Source: CAD feature listing. Evaluate the final solid. Frame: model axes, mm. Coordinates: 2 decimals unless noted, no trailing zeros. Order: outer loops, then holes, each group sorted by start corner. A loop starts at its lowest first (then second) coordinate and runs counter-clockwise, first axis right, second up. Notation, with made-up numbers: (85, 72.5) -> (134, 72.5) arc R10 cw to (134, 89.5) -> close; hole circle Ø6 at (46, -3). An arc over 180 degrees is marked (long way). Put each result on its own line as item: value.
from build123d import *

# Parameters (mm, degrees)
SKETCH1_W            = 40
SKETCH1_H            = 20
BOSS_EXTRUDE1_DEPTH  = 2
M3_CLEARANCE_HOLE1_D = 3.2
FILLET1_R            = 2


with BuildPart() as part:
    # Sketch1 → Boss-Extrude1 (new body)
    with BuildSketch(Plane.XY):
        Rectangle(SKETCH1_W, SKETCH1_H)
    extrude(amount=BOSS_EXTRUDE1_DEPTH)

    # M3 Clearance Hole1 (through all)
    with Locations(Plane.XY.offset(2)):
        with Locations((17.5, -5), (-17.5, 5), (-17.5, -5), (17.5, 5), (0, 5), (0, -5)):
            Hole(M3_CLEARANCE_HOLE1_D / 2)

    # Fillet1
    fillet1_edges = [part.edges().sort_by_distance(p)[0] for p in [
        (20, -10, 1),
        (-20, -10, 1),
        (-20, 10, 1),
        (20, 10, 1),
    ]]
    fillet(fillet1_edges, radius=FILLET1_R)


solid = part.part
1. Ray query, line 1 along Y through (x, z) = (-17.5, 1.05); line 2 along Y through (x, z) = (-0.5, 0.2); line 3 along X through (y, z) = (4.5, 0.6). Return the intervals inside material, ascending.
Numbers:
line 1: y = -10 to -6.6, -3.4 to 3.4, 6.6 to 10
line 2: y = -10 to -6.52, -3.48 to 3.48, 6.52 to 10
line 3: x = -20 to -19.02, -15.98 to -1.52, 1.52 to 15.98, 19.02 to 20
2. Cut plane A-A on x = 0. Output: boundary loops of the cut face in (y, z).
Numbers:
outline: (-10, 0) -> (-6.6, 0) -> (-6.6, 2) -> (-10, 2) -> close; (-3.4, 0) -> (3.4, 0) -> (3.4, 2) -> (-3.4, 2) -> close; (6.6, 0) -> (10, 0) -> (10, 2) -> (6.6, 2) -> close
3. Pull-direction query (X, two-part tool) for faces 1 (the flat face through (20, 0, 1)), 2 (the cylindrical face through (0.35, -6.56, 0.99)), 3 (the flat face through (0, 0, 0)), 4 (the cylindrical face through (-19.43, -9.4, 1.01)); classes: pulls with the +X half, pulls with the -X half, needs draft (parallel to the pull), parting line crosses it, or undercut.
Numbers:
face 1: pulls with the +X half
face 2: undercut
face 3: needs draft
face 4: pulls with the -X half
4. Cut plane B-B on z = 0.75. Output: boundary loops of the cut face in (x, y), plus the area to 3 significant figures.
Numbers:
outline: (-20, -8) arc R2 ccw to (-18, -10) -> (18, -10) arc R2 ccw to (20, -8) -> (20, 8) arc R2 ccw to (18, 10) -> (-18, 10) arc R2 ccw to (-20, 8) -> close; hole circle Ø3.2 at (-17.5, -5); hole circle Ø3.2 at (-17.5, 5); hole circle Ø3.2 at (0, -5); hole circle Ø3.2 at (0, 5); hole circle Ø3.2 at (17.5, -5); hole circle Ø3.2 at (17.5, 5)
area: 748 mm2
5. Cut plane C-C on y = -5. Output: boundary loops of the cut face in (x, z), plus the area to 3 significant figures.
Numbers:
outline: (-20, 0) -> (-19.1, 0) -> (-19.1, 2) -> (-20, 2) -> close; (-15.9, 0) -> (-1.6, 0) -> (-1.6, 2) -> (-15.9, 2) -> close; (1.6, 0) -> (15.9, 0) -> (15.9, 2) -> (1.6, 2) -> close; (19.1, 0) -> (20, 0) -> (20, 2) -> (19.1, 2) -> close
area: 60.8 mm2
